```python
from build123d import *

# Parameters (mm, degrees)
MODEL_R             = 2.45745
MODEL_R_2           = 3.96875
BOSS_EXTRUDE1_DEPTH = 19.05
CUT_EXTRUDE1_REACH  = 843.816
SKETCH2_R           = 2.5527
CUT_EXTRUDE2_REACH  = 843.816
SKETCH4_R           = 2.5527


with BuildPart() as part:
    # Model → Boss-Extrude1 (new body)
    with BuildSketch(Plane.XY):
        with BuildLine():
            Line((785.524844282, 413.072749717), (433.09984428, 413.072749717))
            ThreePointArc((433.09984428, 413.072749717), (424.119588159, 409.353005838), (420.39984428, 400.372749717))
            Line((420.39984428, 400.372749717), (420.39984428, 374.972749717))
            ThreePointArc((420.39984428, 374.972749717), (424.119588159, 365.992493596), (433.09984428, 362.272749717))
            Line((433.09984428, 362.272749717), (452.14984428, 362.272749717))
            ThreePointArc((452.14984428, 362.272749717), (470.110356522, 354.833261959), (477.54984428, 336.872749717))
            Line((477.54984428, 336.872749717), (477.54984428, 222.572749717))
            ThreePointArc((477.54984428, 222.572749717), (470.110356522, 204.612237475), (452.14984428, 197.172749717))
            Line((452.14984428, 197.172749717), (433.09984428, 197.172749717))
            ThreePointArc((433.09984428, 197.172749717), (424.119588159, 193.453005838), (420.39984428, 184.472749717))
            Line((420.39984428, 184.472749717), (420.39984428, 159.072749717))
            ThreePointArc((420.39984428, 159.072749717), (424.119588159, 150.092493596), (433.09984428, 146.372749717))
            Line((433.09984428, 146.372749717), (674.399844282, 146.372749717))
            ThreePointArc((674.399844282, 146.372749717), (683.380100403, 150.092493596), (687.099844282, 159.072749717))
            Line((687.099844282, 159.072749717), (687.099844282, 184.472749717))
            ThreePointArc((687.099844282, 184.472749717), (683.380100403, 193.453005838), (674.399844282, 197.172749717))
            ThreePointArc((674.399844282, 197.172749717), (642.968947858, 210.191853293), (629.949844282, 241.622749717))
            Line((629.949844282, 241.622749717), (629.949844282, 273.372749717))
            ThreePointArc((629.949844282, 273.372749717), (648.548563677, 318.274030322), (693.449844282, 336.872749717))
            Line((693.449844282, 336.872749717), (785.524844282, 336.872749717))
            ThreePointArc((785.524844282, 336.872749717), (794.505100403, 340.592493596), (798.224844282, 349.572749717))
            Line((798.224844282, 349.572749717), (798.224844282, 400.372749717))
            ThreePointArc((798.224844282, 400.372749717), (794.505100403, 409.353005838), (785.524844282, 413.072749717))
        make_face()
        with Locations(Location((518.749844327, 171.772749712, 0), (0, 0, 180))):
            Circle(MODEL_R, mode=Mode.SUBTRACT)
        with Locations(Location((588.526419084, 211.772749722, 0), (0, 0, 180))):
            Circle(MODEL_R, mode=Mode.SUBTRACT)
        with Locations(Location((518.749844281, 260.672749712, 0), (0, 0, 180))):
            Circle(MODEL_R, mode=Mode.SUBTRACT)
        with Locations(Location((588.749844281, 300.672749722, 0), (0, 0, 180))):
            Circle(MODEL_R, mode=Mode.SUBTRACT)
        with Locations(Location((782.349844282, 368.616847103, 0), (0, 0, 180))):
            Circle(MODEL_R_2, mode=Mode.SUBTRACT)
        with Locations(Location((642.649844285, 171.772749717, 0), (0, 0, 180))):
            Circle(MODEL_R, mode=Mode.SUBTRACT)
        with Locations(Location((464.849844282, 171.772749717, 0), (0, 0, 180))):
            Circle(MODEL_R, mode=Mode.SUBTRACT)
        with Locations(Location((464.849844282, 387.672749714, 0), (0, 0, 180))):
            Circle(MODEL_R, mode=Mode.SUBTRACT)
        with Locations(Location((642.649844282, 387.672749714, 0), (0, 0, 180))):
            Circle(MODEL_R, mode=Mode.SUBTRACT)
        with Locations(Location((518.749844281, 300.672749722, 0), (0, 0, 180))):
            Circle(MODEL_R, mode=Mode.SUBTRACT)
        with Locations(Location((588.749844281, 260.672749712, 0), (0, 0, 180))):
            Circle(MODEL_R, mode=Mode.SUBTRACT)
        with Locations(Location((518.749844327, 211.772749722, 0), (0, 0, 180))):
            Circle(MODEL_R, mode=Mode.SUBTRACT)
        with Locations(Location((588.749844281, 171.996174909, 0), (0, 0, 180))):
            Circle(MODEL_R, mode=Mode.SUBTRACT)
        with BuildLine():
            ThreePointArc((444.9702071, 177.167541541), (444.259969282, 171.772749717), (444.9702071, 166.377957893))
            ThreePointArc((444.9702071, 166.377957893), (441.568935094, 160.486781969), (435.677759169, 163.888053974))
            ThreePointArc((435.677759169, 163.888053974), (434.639719282, 171.772749717), (435.677759169, 179.657445459))
            ThreePointArc((435.677759169, 179.657445459), (441.568935094, 183.058717465), (444.9702071, 177.167541541))
        make_face(mode=Mode.SUBTRACT)
        with BuildLine():
            ThreePointArc((671.821929397, 163.888053974), (672.859969285, 171.772749717), (671.821929397, 179.657445459))
            ThreePointArc((671.821929397, 179.657445459), (665.930753473, 183.058717465), (662.529481467, 177.167541541))
            ThreePointArc((662.529481467, 177.167541541), (663.239719285, 171.772749717), (662.529481467, 166.377957893))
            ThreePointArc((662.529481467, 166.377957893), (665.930753473, 160.486781969), (671.821929397, 163.888053974))
        make_face(mode=Mode.SUBTRACT)
        with BuildLine():
            ThreePointArc((671.821929395, 379.788053972), (672.859969282, 387.672749714), (671.821929395, 395.557445457))
            ThreePointArc((671.821929395, 395.557445457), (665.93075347, 398.958717463), (662.529481465, 393.067541538))
            ThreePointArc((662.529481465, 393.067541538), (663.239719282, 387.672749714), (662.529481465, 382.277957891))
            ThreePointArc((662.529481465, 382.277957891), (665.93075347, 376.386781966), (671.821929395, 379.788053972))
        make_face(mode=Mode.SUBTRACT)
        with BuildLine():
            ThreePointArc((444.9702071, 393.067541538), (444.259969282, 387.672749714), (444.9702071, 382.277957891))
            ThreePointArc((444.9702071, 382.277957891), (441.568935094, 376.386781966), (435.677759169, 379.788053972))
            ThreePointArc((435.677759169, 379.788053972), (434.639719282, 387.672749714), (435.677759169, 395.557445457))
            ThreePointArc((435.677759169, 395.557445457), (441.568935094, 398.958717463), (444.9702071, 393.067541538))
        make_face(mode=Mode.SUBTRACT)
    extrude(amount=BOSS_EXTRUDE1_DEPTH)

    # Sketch2 → Cut-Extrude1 (cut, up to next)
    with BuildSketch(Plane.XZ.offset(-146.372749717), mode=Mode.PRIVATE) as cut_extrude1_sk1:
        with Locations(Location((439.83084428, 9.525, 0), (0, 0, 270))):
            Circle(SKETCH2_R)
    cut_extrude1_tool1 = extrude(cut_extrude1_sk1.sketch, amount=-CUT_EXTRUDE1_REACH, mode=Mode.PRIVATE) & part.part
    # Sketch2 → Cut-Extrude1 (cut, up to next)
    with BuildSketch(Plane.XZ.offset(-146.372749717), mode=Mode.PRIVATE) as cut_extrude1_sk2:
        with Locations(Location((667.668844282, 9.525, 0), (0, 0, 270))):
            Circle(SKETCH2_R)
    cut_extrude1_tool2 = extrude(cut_extrude1_sk2.sketch, amount=-CUT_EXTRUDE1_REACH, mode=Mode.PRIVATE) & part.part
    add(cut_extrude1_tool1.solids().sort_by_distance((439.830844, 146.37275, 9.525))[0], mode=Mode.SUBTRACT)
    add(cut_extrude1_tool2.solids().sort_by_distance((667.668844, 146.37275, 9.525))[0], mode=Mode.SUBTRACT)

    # Sketch4 → Cut-Extrude2 (cut, up to next)
    with BuildSketch(Plane(origin=(0, 413.072749717, 0), x_dir=(1, 0, 0), z_dir=(0, 1, 0)), mode=Mode.PRIVATE) as cut_extrude2_sk1:
        with Locations(Location((439.83084428, -9.525, 0), (0, 0, 90))):
            Circle(SKETCH4_R)
    cut_extrude2_tool1 = extrude(cut_extrude2_sk1.sketch, amount=-CUT_EXTRUDE2_REACH, mode=Mode.PRIVATE) & part.part
    # Sketch4 → Cut-Extrude2 (cut, up to next)
    with BuildSketch(Plane(origin=(0, 413.072749717, 0), x_dir=(1, 0, 0), z_dir=(0, 1, 0)), mode=Mode.PRIVATE) as cut_extrude2_sk2:
        with Locations(Location((667.668844282, -9.525, 0), (0, 0, 90))):
            Circle(SKETCH4_R)
    cut_extrude2_tool2 = extrude(cut_extrude2_sk2.sketch, amount=-CUT_EXTRUDE2_REACH, mode=Mode.PRIVATE) & part.part
    add(cut_extrude2_tool1.solids().sort_by_distance((439.830844, 413.07275, 9.525))[0], mode=Mode.SUBTRACT)
    add(cut_extrude2_tool2.solids().sort_by_distance((667.668844, 413.07275, 9.525))[0], mode=Mode.SUBTRACT)


solid = part.part
```
Here's how the part is built. I have some questions about the finished solid (model axes, mm). A direction names the side the tool comes from. Give positions to 0.01 mm unless a question says otherwise; leave off trailing zeros. Loops run counter-clockwise (first coordinate to the right, second up) from the corner with the lowest first, then second, coordinate; pieces in that order, holes last. Notation, with made-up numbers: M -37,-14.5 L 5,-14.5 A18 cw 5,12.5 Z; hole C 34,74.5 d11. An arc over 180 degrees is marked long. Use one line per item in the form item = value. Start each with the question number.
Q1. If we section it at A-A (x = 652.5): Write out the boundary of the cut face in (y, z).
Q2. If we section it at D-D (y = 231.5): Write out the boundary of the cut face in (x, z).
Q3. If we section it at C-C (z = 15.75): State how many separate pieces and enclosed holes the cut face has, then the cut area to 3 significant figures.
Q4. Will these pins go through, and if not, where does the flat tip stop? pin 1 Ø6 at (y, z) = (221.5, 5.5) entering from +X; pin 2 Ø3 at (x, z) = (439.83, 9.52) entering from -Y; pin 3 Ø4 at (x, z) = (667.67, 9.52) entering from +Y; pin 4 Ø4 at (x, y) = (464.85, 387.67) entering from +Z.
Q5. Which directions (+Z, -Z, +X, -X, +Y, -Y) give clear straight access to the entire face, cutting with the end or side of a thin tool? Please do faces 4 (the cylindrical face through (794.406, 340.494, 9.392)), 5 (the flat face through (629.95, 257, 9)), 6 (the cylindrical face through (434.64, 387.56, 9.39)), 7 (the cylindrical face through (469.91, 355.03, 9.39)).
Q6. I need wall thicknesses on line 1 along X through (y, z) = (387.5, 1.5); line 2 along Y through (x, z) = (735.5, 9); line 3 along X through (y, z) = (167.5, 3). Which ranges of each line are inside material? Lowest first, please.
Q7. Thinking about a two-plate mould opening in X: for faces 1 (the cylindrical face through (424.021, 150.192, 9.392)), 2 (the cylindrical face through (663.24, 387.75, 9.39)), 3 (the cylindrical face through (683.48, 193.35, 9.39)), which applies, +X half, -X half, draft (parallel to the pull), parting line (faces both ways), or undercut?
Q8. If we section it at B-B (x = 760): Write out the boundary of the cut face in (y, z), then the cut area to 3 significant figures.
Taken from the geometry:
q1.outline = M 146.37,0 L 202.94,0 L 202.94,19.05 L 146.37,19.05 Z; M 321.9,0 L 413.07,0 L 413.07,19.05 L 321.9,19.05 Z
q2.outline = M 477.55,0 L 631.12,0 L 631.12,19.05 L 477.55,19.05 Z
q3.separate_pieces = 1
q3.enclosed_holes = 17
q3.area = 62,400 mm^2
q4.pin_1 = 636.44
q4.pin_2 = 182.79
q4.pin_3 = 376.92
q4.pin_4 = through
q5.face_4 = +Z, -Z, +X, -Y
q5.face_5 = +Z, -Z, +X
q5.face_6 = +Z, -Z
q5.face_7 = +Z, -Z, -X
q6.line_1 = 420.4 to 434.64, 444.26 to 462.4, 467.3 to 640.2, 645.1 to 663.24, 672.86 to 798.22
q6.line_2 = 336.87 to 413.07
q6.line_3 = 420.4 to 434.94, 444.7 to 662.8, 672.56 to 687.1
q7.face_1 = -X half
q7.face_2 = undercut
q7.face_3 = +X half
q8.outline = M 336.87,0 L 413.07,0 L 413.07,19.05 L 336.87,19.05 Z
q8.area = 1,450 mm^2
